Autodesk Inventor part; units mm, degrees
ref_plane "YZ Plane" through (0, 0, 0) normal (1, 0, 0) x (0, 1, 0)
ref_plane "XZ Plane" through (0, 0, 0) normal (0, 1, 0) x (-1, 0, 0)
ref_plane "XY Plane" through (0, 0, 0) normal (0, 0, 1) x (1, 0, 0)
sketch "Эскиз1" plane through (0, 0, 0) normal (0, 0, 1) x (1, 0, 0)
  line L0 (0, 0) -> (0, 20)
  line L1 (0, 20) -> (2.8284, 22.8284)
  line L2 (0, 0) -> (15, 0)
  line L3 (15, 0) -> (15, 20)
  line L4 (15, 20) -> (12.1716, 22.8284)
  line L5 (12.1716, 22.8284) -> (2.8284, 22.8284)
  dimension "d0" = 20
  dimension "d1" = 4
  dimension "d2" = 135
  dimension "d3" = 15
  dimension "d4" = 4
  dimension "d5" = 135
revolve "Вращение1" add sketch "Эскиз1" angle 360 about axis through (0, 0, 0) along (1, 0, 0)
sketch "Эскиз2" plane through (0, 0, 0) normal (-1, 0, 0) x (0, 0, 1)
  circle A0 centre (0, 16) radius 1.75
  point P0 (0, 0)
  dimension "d7" = 3.5
  dimension "d8" = 16
extrude "Выдавливание1" cut sketch "Эскиз2" against normal blind 15
sketch "Эскиз3" plane through (0, 0, 0) normal (0, 1, 0) x (-1, 0, 0)
  line L0 (-15, 20) -> (-15, -20) construction
  line L1 (-15, 0) -> (-8, 0)
  line L2 (-8, 0) -> (-8, -10)
  line L3 (-8, -10) -> (-15, -10)
  line L4 (-15, -10) -> (-15, 0)
  point P0 (0, 0)
  dimension "d11" = 7
  dimension "d12" = 10
revolve "Вращение2" cut sketch "Эскиз3" angle 360 about axis through (15, 0, 0) along (-1, 0, 0)
properties part number "711122"
Part model, mm, in its own coordinate system. A direction names the side the tool comes from. Round coordinates to 2 decimals unless told otherwise and drop trailing zeros. Write each loop counter-clockwise with the first axis right and the second up, starting at its lowest first coordinate (ties: lowest second). Pieces come first, ordered by that corner, then holes.
Item 1: Two-plate mould, pull along Y, no slides. Class faces 1 (the conical face through (14.82, -16.01, 12.28)), 2 (the flat face through (0, 0, 0)), 3 (the cylindrical face through (7.395, 17.735, -0.228)): +Y half, -Y half, draft (parallel to the pull), parting line (faces both ways), or undercut.
Results:
face 1: parting line
face 2: draft
face 3: undercut
Item 2: Which spindle directions (+Z, -Z, +X, -X, +Y, -Y) get a long thin tool onto all of the face, cutting with end or side? Do faces 4 (the cylindrical face through (11.55, -9.76, 2.17)), 5 (the conical face through (0.18, -2.63, 20.01)). Say none if no direction does.
Results:
face 4: +X
face 5: -X
Item 3: Drop flat-ended pins along their axis: pin 1 Ø3 at (x, y) = (9, -11.5) entering from +Z; pin 2 Ø8 at (x, z) = (4, -9.5) entering from +Y; pin 3 Ø3 at (y, z) = (11.5, -6) entering from -X; pin 4 Ø2 at (x, z) = (3, 12) entering from -Y. Give the stop position or say it passes through.
Results:
pin 1: stops at z = 20.52
pin 2: stops at y = 22.16
pin 3: stops at x = 0
pin 4: stops at y = -20
Item 4: Probe L1, parallel to Y at x = 9, z = 1.5; L2, parallel to Z at x = 10.5, y = 0; L3, parallel to Y at x = 11.25, z = 1. List the from-to ranges inside material, lowest first.
Results:
L1: y = -22.78 to -9.89, 9.89 to 15.1, 16.9 to 22.78
L2: z = -22.83 to -10, 10 to 22.83
L3: y = -22.81 to -9.95, 9.95 to 14.56, 17.44 to 22.81
Item 5: Cut at B-B, the plane y = 0. Give the cut face in (x, z), plus the area to 3 significant figures.
Results:
outline: (0, -20) - (2.83, -22.83) - (12.17, -22.83) - (15, -20) - (15, -10) - (8, -10) - (8, 10) - (15, 10) - (15, 20) - (12.17, 22.83) - (2.83, 22.83) - (0, 20) - close
area: 529 mm2
Item 6: Cut at A-A, the plane z = 0. Give the cut face in (x, y).
Results:
outline: (0, -20) - (2.83, -22.83) - (12.17, -22.83) - (15, -20) - (15, -10) - (8, -10) - (8, 10) - (15, 10) - (15, 14.25) - (0, 14.25) - close; (0, 17.75) - (15, 17.75) - (15, 20) - (12.17, 22.83) - (2.83, 22.83) - (0, 20) - close
Item 7: Cut at C-C, the plane x = 4.25. Give the cut face in (y, z), plus the area to 3 significant figures.
Results:
outline: circle Ø45.66 at (0, 0); hole circle Ø3.5 at (16, 0)
area: 1,630 mm2
